Answer from the drawing. Dimensions are ordinates in mm from the lowest x, y and z of the part. A direction names the side the tool comes from. Coordinates: 2 decimals unless noted, no trailing zeros. Write each loop counter-clockwise with the first axis right and the second up, starting at its lowest first coordinate (ties: lowest second). Pieces come first, ordered by that corner, then holes. Notation, with made-up numbers: (-33, 26.25) - (-24, 26.25) arc R22 ccw to (-24, 65.25) - close; hole circle Ø3 at (57.5, -13.75). An arc over 180 degrees is marked (long way). Use CSV: the item, a comma, the result in double quotes. Start each with the question number.
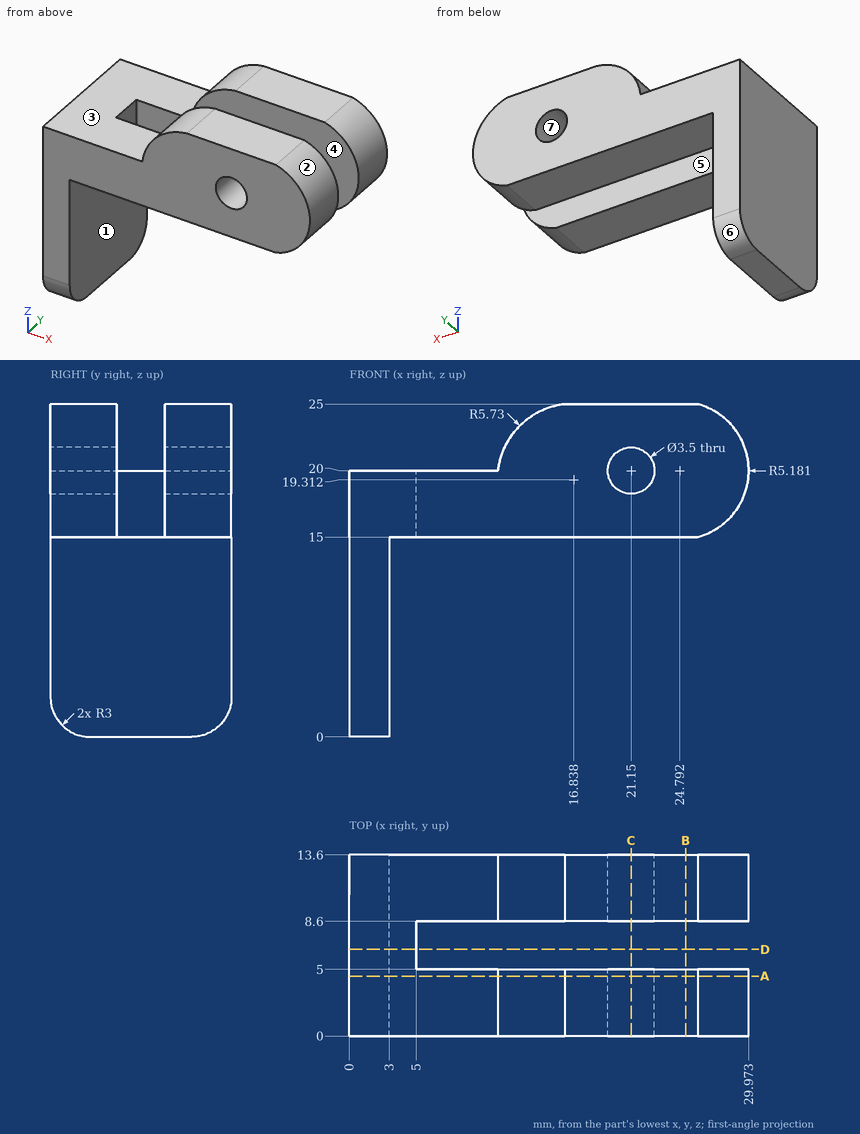
Item 1: Each of these flat-tipped pins is pushed along its axis until it touches: pin 1 (3.5 mm diameter, centred on x = 5, y = 7, fed in from +Z); pin 2 (8 mm diameter, centred on x = 12, y = 6, fed in from -Z); pin 3 (5 mm diameter, centred on y = 1.5, z = 21, fed in from -X); pin 4 (4 mm diameter, centred on y = 7, z = 18.5, fed in from +X). Where does it stop, or does it pass through?
Item 2: Determine the mould class of the marked faces 4, 5, 6 and 7 for opening direction Y: +Y half, -Y half, draft (parallel to the pull), parting line (faces both ways), or undercut.
Item 3: A cutting plane is placed at C-C (x = 21.15). Determine the outline of the cut face in (y, z), then the cut area to 3 significant figures.
Item 4: Which of the six approach directions +Z, -Z, +X, -X, +Y, -Y give full straight-line access (tool end or side, diameter ignored) to the marked faces 1, 2 and 3?
Item 5: A cutting plane is placed at D-D (y = 6.5). Determine the outline of the cut face in (x, z).
Item 6: Straight lines are drawn through the part: probe 1 along Y at (x, z) = (14.75, 16.5); probe 2 along Z at (x, y) = (17.25, 10.25); probe 3 along Z at (x, y) = (8.25, 4.5). For each, find the intervals that lie inside material, in ascending order. Write a range as [from, to].
Item 7: A cutting plane is placed at A-A (y = 4.5). Determine the outline of the cut face in (x, z).
Item 8: A cutting plane is placed at B-B (x = 25.25). Determine the outline of the cut face in (y, z).
Calculated:
1,pin 1,"stops at z = 20"
1,pin 2,"stops at z = 15"
1,pin 3,"stops at x = 0"
1,pin 4,"stops at x = 29.96"
2,face 4,"undercut"
2,face 5,"undercut"
2,face 6,"+Y half"
2,face 7,"draft"
3,outline,"(0, 15) - (5, 15) - (5, 18.25) - (0, 18.25) - close; (0, 21.75) - (5, 21.75) - (5, 25) - (0, 25) - close; (8.6, 15) - (13.6, 15) - (13.6, 18.25) - (8.6, 18.25) - close; (8.6, 21.75) - (13.6, 21.75) - (13.6, 25) - (8.6, 25) - close"
3,area,"65.0 mm²"
4,face 1,"-Z, +X, +Y, -Y"
4,face 2,"+X, +Y, -Y"
4,face 3,"+Z, -X, +Y, -Y"
5,outline,"(0, 0) - (3, 0) - (3, 15) - (5, 15) - (5, 20) - (0, 20) - close"
6,probe 1,"y = [0, 5], [8.6, 13.6]"
6,probe 2,"z = [15, 25]"
6,probe 3,"z = [15, 20]"
7,outline,"(0, 0) - (3, 0) - (3, 15) - (26.15, 15) arc R5.18 ccw to (26.15, 25) - (16.15, 25) arc R5.73 ccw to (11.15, 20) - (0, 20) - close; hole circle Ø3.5 at (21.15, 20)"
8,outline,"(0, 15) - (5, 15) - (5, 25) - (0, 25) - close; (8.6, 15) - (13.6, 15) - (13.6, 25) - (8.6, 25) - close"
